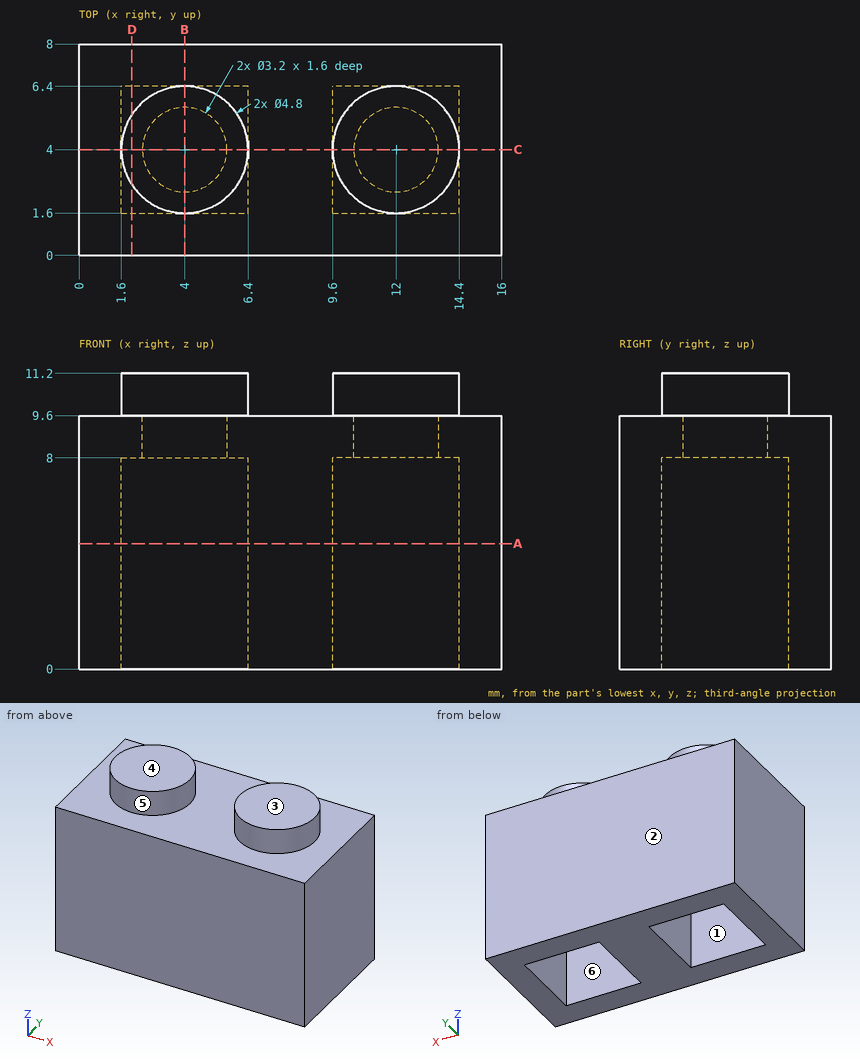
Source: three-view drawing plus pictorial views. Frame: mm from the lowest corner of the part. A direction names the side the tool comes from. Give positions to 0.01 mm unless a question says otherwise; leave off trailing zeros. Order: outer loops, then holes, each group sorted by start corner. A loop starts at its lowest first (then second) coordinate and runs counter-clockwise, first axis right, second up. Notation, with made-up numbers: (-11.75, 40) -> (35.25, 40) arc R31 cw to (35.25, 66) -> close; hole circle Ø8 at (63.25, 72.25). An arc over 180 degrees is marked (long way). Write each question's results on one line, items separated by ' | '. Start each with the question number.
Item 1: Cut plane D-D on x = 2. Return the cut outline in (y, z).
Item 2: Set-up query: the marked faces 4, 5 and 6. Return all of +Z, -Z, +X, -X, +Y, -Y with unobstructed straight access to the full face (end or side cutting, diameter ignored); none if empty.
Item 3: Cut plane C-C on y = 4. Return the cut outline in (x, z), then the cut area to 3 significant figures.
Item 4: Cut plane B-B on x = 4. Return the cut outline in (y, z), then the cut area to 3 significant figures.
Item 5: Cut plane A-A on z = 4.75. Return the cut outline in (x, y).
Item 6: Mould query, pull axis Y, two halves, no side actions, for the marked faces 1, 2 and 3. Classes: pulls with the +Y half, pulls with the -Y half, needs draft (parallel to the pull), parting line crosses it, or undercut.
Item 7: Line query: line 1 (X direction, y = 5.25, z = 6.5); line 2 (Y direction, x = 12, z = 8.65); line 3 (Y direction, x = 5.75, z = 6.75). Output: solid intervals per line, ascending.
Item 8: Contact query for flat-ended pins moving along their axis: P1, Ø3.5, axis at x = 3.5, y = 4.5, coming from the -Z side; P2, Ø2.5, axis at x = 12, y = 4, coming from the -Z side. Output: stop coordinate, or through.
Established:
1) outline: (0, 0) -> (1.6, 0) -> (1.6, 8) -> (6.4, 8) -> (6.4, 0) -> (8, 0) -> (8, 9.6) -> (5.33, 9.6) -> (5.33, 11.2) -> (2.67, 11.2) -> (2.67, 9.6) -> (0, 9.6) -> close
2) face 4: +Z, +X, -X, +Y, -Y | face 5: +Z | face 6: -Z
3) outline: (0, 0) -> (1.6, 0) -> (1.6, 8) -> (2.4, 8) -> (2.4, 9.6) -> (5.6, 9.6) -> (5.6, 8) -> (6.4, 8) -> (6.4, 0) -> (9.6, 0) -> (9.6, 8) -> (10.4, 8) -> (10.4, 9.6) -> (13.6, 9.6) -> (13.6, 8) -> (14.4, 8) -> (14.4, 0) -> (16, 0) -> (16, 9.6) -> (14.4, 9.6) -> (14.4, 11.2) -> (9.6, 11.2) -> (9.6, 9.6) -> (6.4, 9.6) -> (6.4, 11.2) -> (1.6, 11.2) -> (1.6, 9.6) -> (0, 9.6) -> close | area: 81.9 mm^2
4) outline: (0, 0) -> (1.6, 0) -> (1.6, 8) -> (2.4, 8) -> (2.4, 9.6) -> (5.6, 9.6) -> (5.6, 8) -> (6.4, 8) -> (6.4, 0) -> (8, 0) -> (8, 9.6) -> (6.4, 9.6) -> (6.4, 11.2) -> (1.6, 11.2) -> (1.6, 9.6) -> (0, 9.6) -> close | area: 41.0 mm^2
5) outline: (0, 0) -> (16, 0) -> (16, 8) -> (0, 8) -> close; hole (1.6, 1.6) -> (6.4, 1.6) -> (6.4, 6.4) -> (1.6, 6.4) -> close; hole (9.6, 1.6) -> (14.4, 1.6) -> (14.4, 6.4) -> (9.6, 6.4) -> close
6) face 1: undercut | face 2: pulls with the +Y half | face 3: needs draft
7) line 1: 0 to 1.6, 6.4 to 9.6, 14.4 to 16 | line 2: 0 to 2.4, 5.6 to 8 | line 3: 0 to 1.6, 6.4 to 8
8) P1: z = 8 | P2: z = 9.6
